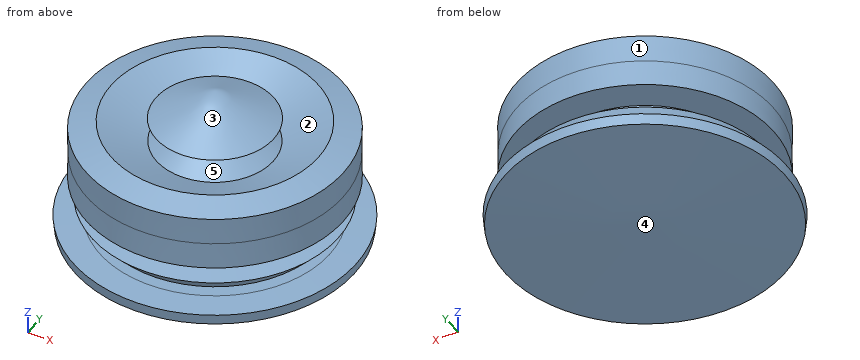
from build123d import *


with BuildPart() as f1:
    # F0 (on Front) → F1 (revolve)
    with BuildSketch(Plane.XZ):
        Polygon((29.873788, 61.614744), (0, 76.759115), (0, 0), (70.9503, 1.867101), (71.572691, 7.260978), (58.295429, 7.675901), (39.209366, 7.053524), (27.591765, 7.675901), (14.521956, 11.410132), (11.617556, 19.293495), (39.001912, 13.277248), (54.976106, 10.165378), (62.444568, 18.25621), (46.26292, 21.16061), (49.997151, 29.04398), (65.141499, 28.836526), (64.934045, 42.321235), (65.141499, 56.220867), (52.486628, 59.95509), (29.666334, 48.959866), (10.787725, 61.614744), align=None)
    revolve(axis=Axis((0, 0, 38.379557), (0, 0, 1)))


solid = f1.part
Could you check a few things on this model? Use its own coordinates, in mm. Face numbers are marked on the shaded views. A direction names the side the tool comes from. Give positions to 0.01 mm unless a question says otherwise; leave off trailing zeros. Write each loop counter-clockwise with the first axis right and the second up, starting at its lowest first coordinate (ties: lowest second). Pieces come first, ordered by that corner, then holes. Notation, with made-up numbers: (88, 76.25) -> (95, 76.25) arc R27 cw to (95, 102.25) -> close; hole circle Ø3 at (41, -29). An arc over 180 degrees is marked (long way). Write each question's results on one line, items separated by ' | '. Start each with the question number.
Q1. I need wall thicknesses on probe 1 along Z at (x, y) = (-24, -6.5); probe 2 along X at (y, z) = (5.5, 56); probe 3 along Z at (x, y) = (42.5, 28.5). Which ranges of each line are inside material? Lowest first, please.
Q2. We'd pull the mould along X, two halves only. Please class the marked faces 1 and 2: +X half, -X half, draft (parallel to the pull), parting line (faces both ways), or undercut.
Q3. I'm going to push flat-ended pins straight in: pin 1 Ø10 at (x, y) = (0.5, -48.5) entering from -Z; pin 2 Ø1.5 at (x, z) = (-4.5, 53.5) entering from -Y; pin 3 Ø10 at (x, y) = (16.5, -44) entering from +Z. Where does each tip first touch, or does it pass through?
Q4. Which directions (+Z, -Z, +X, -X, +Y, -Y) give clear straight access to the entire face, cutting with the end or side of a thin tool? Please do the marked faces 3, 4 and 5.
Q5. Suppose I cut it at A-A, the plane x = 19. State how many separate pieces and enclosed holes the cut face has, and give its area (3 significant figures).
Q6. Suppose I cut it at C-C, the plane z = 72. List the corners of the cut face in (x, y) for me.
Outcome:
1) probe 1: 0.65 to 8.46, 16.38 to 52.18, 61.61 to 64.15 | probe 2: -64.91 to -43.94, -18.36 to 18.36, 43.94 to 64.91 | probe 3: 1.35 to 7.44, 10.91 to 20.28, 29.03 to 59.32
2) face 1: parting line | face 2: undercut
3) pin 1: z = 1.14 | pin 2: y = -64.99 | pin 3: z = 59.72
4) face 3: +Z | face 4: -Z | face 5: none
5) separate pieces: 3 | enclosed holes: 0 | area: 5,750 mm2
6) outline: circle Ø18.78 at (0, 0)
